Part model, mm, in its own coordinate system. Give positions to 0.01 mm unless a question says otherwise; leave off trailing zeros. Write each loop counter-clockwise with the first axis right and the second up, starting at its lowest first coordinate (ties: lowest second). Pieces come first, ordered by that corner, then holes. Notation, with made-up numbers: M -3.75,-5.5 L 24.25,-5.5 A21 ccw 24.25,29.5 Z; hole C -34.75,20.25 d3. An arc over 180 degrees is marked long. Use a Markdown table: item, result.
```python
from build123d import *

# Parameters (mm, degrees)
F0_R          = 26.2972038965
F0_R_2        = 21.7596703079
F1_DEPTH      = 25.4
F2_DEPTH      = 25.4
F3_DEPTH      = 50.801
F3_DEPTH_BACK = 310.4061427


# Not quite as in the source:
# - an extrude ends at something that could not be found from the text; its depth is read off the source's solid
# - a feature of the source that left no trace in its solid (it failed there, or was rolled back) is left out
# - a pattern or mirror of a feature is missing from the dataset's text; its kind, count and spacing are read off the source's solid


with BuildPart() as f1:
    # F0 (on Front) → F1 (new body)
    with BuildSketch(Plane.XZ):
        with Locations((35.550635308, 42.1431325376)):
            Circle(F0_R)
        with Locations((35.550635308, 42.1431325376)):
            Circle(F0_R_2, mode=Mode.SUBTRACT)
        with Locations((35.550635308, 42.1431325376)):
            Circle(F0_R_2)
    extrude(amount=-F1_DEPTH)

    # F2 (add): a face of the model
    f2_faces = [f1.faces().sort_by_distance(p)[0] for p in [
        (35.550635308, 0, 42.1431325376),
    ]]
    extrude(f2_faces, amount=F2_DEPTH)

    # F3 (add, two sides): a face of the model
    f3_faces = [f1.faces().sort_by_distance(p)[0] for p in [
        (35.550635308, -25.4, 42.1431325376),
    ]]
    f3 = extrude(f3_faces, amount=-F3_DEPTH) + extrude(f3_faces, amount=F3_DEPTH_BACK)

    # F3_copies: F3 across plane
    add(f3.mirror(Plane.ZX.offset(-135.562021)))


solid = f1.part
```
1. Drill centre lines: L1, parallel to Z at x = 37, y = -6; L2, parallel to X at y = -239.5, z = 43; L3, parallel to X at y = -234, z = 50.5. Where is each one in solid material? Low to high.
Findings below:
| item | result |
|---|---|
| L1 | 15.89 to 68.4 |
| L2 | 9.27 to 61.83 |
| L3 | 10.62 to 60.48 |
2. Cut at C-C, the plane y = -202.5. Give the cut face in (x, z).
Findings below:
| item | result |
|---|---|
| outline | C 35.55,42.14 d52.59 |
3. Drop flat-ended pins along their axis: P1, Ø4, axis at y = -10.5, z = 46.5, coming from the -X side; P2, Ø8, axis at y = -78, z = 43, coming from the +X side; P3, Ø5, axis at x = 52.5, y = -30.5, coming from the +Z side; P4, Ø1.5, axis at y = -222.5, z = 38.5, coming from the +X side. Give the stop position or say it passes through.
Findings below:
| item | result |
|---|---|
| P1 | x = 9.36 |
| P2 | x = 61.85 |
| P3 | z = 64.11 |
| P4 | x = 61.69 |
4. Cut at B-B, the plane x = 55. Give the cut face in (y, z).
Findings below:
| item | result |
|---|---|
| outline | M -335.81,24.44 L 64.68,24.44 L 64.68,59.84 L -335.81,59.84 Z |
5. Cut at A-A, the plane z = 54. Give the cut face in (x, y).
Findings below:
| item | result |
|---|---|
| outline | M 12.08,-335.81 L 59.02,-335.81 L 59.02,64.68 L 12.08,64.68 Z |
